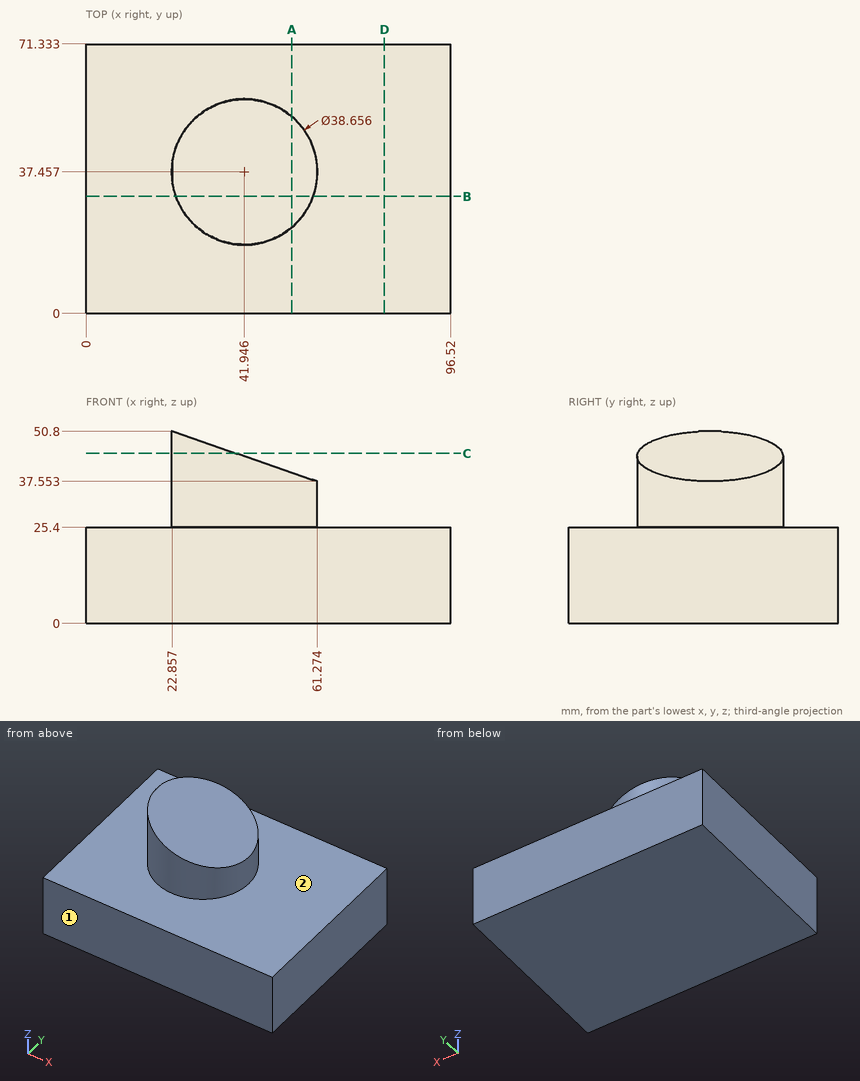
Input: dimensioned drawing with shaded views. Units: mm. Origin: part minimum x, y, z. A direction names the side the tool comes from. Coordinates: 2 decimals unless noted, no trailing zeros. Loops run counter-clockwise (first coordinate to the right, second up) from the corner with the lowest first, then second, coordinate; pieces in that order, holes last.
Q1. Section A-A, the plane x = 54.5. Return the cut outline in (y, z).
Results are:
outline: (0, 0) - (71.33, 0) - (71.33, 25.4) - (52.15, 25.4) - (52.15, 39.89) - (22.76, 39.89) - (22.76, 25.4) - (0, 25.4) - close
Q2. Section B-B, the plane y = 31. Return the cut outline in (x, z).
Results are:
outline: (0, 0) - (96.52, 0) - (96.52, 25.4) - (60.16, 25.4) - (60.16, 37.94) - (23.73, 50.5) - (23.73, 25.4) - (0, 25.4) - close
Q3. Set-up query: the marked faces 1 and 2. Return all of +Z, -Z, +X, -X, +Y, -Y with unobstructed straight access to the full face (end or side cutting, diameter ignored); none if empty.
Results are:
face 1: +Z, -Z, +X, -X, -Y
face 2: +Z
Q4. Section C-C, the plane z = 45. Return the cut outline in (x, y), and give its area (3 significant figures).
Results are:
outline: (39.68, 18.26) - (39.68, 56.65) arc R19.33 ccw to start
area: 499 mm2
Q5. Line query: line 1 along Z through (x, y) = (22.5, 55); line 2 along Y through (x, z) = (30, 35); line 3 along X through (y, z) = (30, 26) (1 decimal). Output: solid intervals per line, ascending.
Results are:
line 1: z = 0 to 25.4
line 2: y = 22.26 to 52.65
line 3: x = 24.1 to 59.8
Q6. Contact query for flat-ended pins moving along their axis: pin 1 (6 mm diameter, centred on x = 47, y = 36.5, fed in from +Z); pin 2 (3 mm diameter, centred on x = 21, y = 63.5, fed in from +Z); pin 3 (12 mm diameter, centred on y = 56.5, z = 44.5, fed in from -X). Output: stop coordinate, or through.
Results are:
pin 1: stops at z = 43.51
pin 2: stops at z = 25.4
pin 3: stops at x = 27.68
Q7. Section D-D, the plane x = 79. Return the cut outline in (y, z).
Results are:
outline: (0, 0) - (71.33, 0) - (71.33, 25.4) - (0, 25.4) - close
